Here's how the part is built. I have some questions about the finished solid (model axes, mm). A direction names the side the tool comes from. Round coordinates to 2 decimals unless told otherwise and drop trailing zeros. Loops run counter-clockwise (first coordinate to the right, second up) from the corner with the lowest first, then second, coordinate; pieces in that order, holes last. Notation, with made-up numbers: (1.25, -12.5) - (20.25, -12.5) arc R21 ccw to (20.25, -0.5) - close; hole circle Ø10 at (-20, 55.25). An arc over 180 degrees is marked (long way). Answer as a JSON object with one key per item and string values. Group by question number.
1) If I drill on line 1 along Y through (x, z) = (-11.5, -27); line 2 along Y through (x, z) = (7.5, 13); line 3 along X through (y, z) = (-6.5, -13.5), over which ranges is the centre line in solid material (lowest first)? Write a range as [from, to].
2) If we mould it in two halves opening along X, with no side actions, what happens to faces 1 (the face through (-15.825, -5, -20)), 2 (the face through (-6, -5, -30)), 3 (the face through (10, -24, -4)), 4 (the face through (-22, -26, -4))? For each: pulls with the +X half, pulls with the -X half, needs draft (parallel to the pull), parting line crosses it, or undercut.
3) I want a section at C-C, the plane y = -46. Please give me the cut outline in (x, z).
4) I want a section at D-D, the plane x = -6. Please give me the cut outline in (y, z).
5) I want a section at B-B, the plane x = -18. Please give me the cut outline in (y, z).
6) Which directions (+Z, -Z, +X, -X, +Y, -Y) give clear straight access to the entire face, cutting with the end or side of a thin tool? Please do faces 5 (the face through (6, -5, -27)), 6 (the face through (-2, -10, -20)), 7 (the face through (-6, -20, 2)).
7) Will these pins go through, and if not, where does the flat tip stop? P1, Ø6, axis at x = -4.5, y = -14.5, coming from the -Z side; P2, Ø5, axis at x = -1, y = -6, coming from the +Z side; P3, Ø8, axis at x = -7, z = -14.5, coming from the +Y side.
8) I want a section at A-A, the plane z = -19.5. Please give me the cut outline in (x, y) (3 decimals), then the cut area to 4 significant figures.
from build123d import *

# Parameters (mm, degrees)
F1_DEPTH = 50
F2_W     = 40
F2_H     = 28
F2_H_2   = 20
F3_DEPTH = 32.001
F4_SIZE  = 1


with BuildPart() as f1:
    # F0 (on Front) → F1 (new body)
    with BuildSketch(Plane.XZ):
        with BuildLine():
            Line((-22, 30), (-22, -30))
            Line((-22, -30), (-2, -30))
            Line((-2, -30), (-2, 9.9960947032))
            ThreePointArc((-2, 9.9960947032), (-8.25, 18), (-2, 26.0039052968))
            Line((-2, 26.0039052968), (-2, 30))
            Line((-2, 30), (-22, 30))
        make_face()
        with BuildLine():
            ThreePointArc((-15.825, -24.825), (-18, -27), (-20.175, -24.825))
            Line((-20.175, -24.825), (-20.175, -15.175))
            ThreePointArc((-20.175, -15.175), (-18, -13), (-15.825, -15.175))
            Line((-15.825, -15.175), (-15.825, -24.825))
        make_face(mode=Mode.SUBTRACT)
        with BuildLine():
            ThreePointArc((-3.825, -24.825), (-6, -27), (-8.175, -24.825))
            Line((-8.175, -24.825), (-8.175, -15.175))
            ThreePointArc((-8.175, -15.175), (-6, -13), (-3.825, -15.175))
            Line((-3.825, -15.175), (-3.825, -24.825))
        make_face(mode=Mode.SUBTRACT)
        with BuildLine():
            Line((-2, 9.9960947032), (-2, -30))
            Line((-2, -30), (10, -30))
            Line((10, -30), (10, 30))
            Line((10, 30), (-2, 30))
            Line((-2, 30), (-2, 26.0039052968))
            ThreePointArc((-2, 26.0039052968), (5.0775240029, 24.5024034018), (8.25, 18))
            ThreePointArc((8.25, 18), (5.0775240029, 11.4975965982), (-2, 9.9960947032))
        make_face()
        with BuildLine():
            Line((3.825, -24.825), (3.825, -15.175))
            ThreePointArc((3.825, -15.175), (6, -13), (8.175, -15.175))
            Line((8.175, -15.175), (8.175, -24.825))
            ThreePointArc((8.175, -24.825), (6, -27), (3.825, -24.825))
        make_face(mode=Mode.SUBTRACT)
    extrude(amount=F1_DEPTH)

    # F2 (on face) → F3 (cut, through all)
    with BuildSketch(Plane.YZ.offset(10)):
        with Locations((-20, 16)):
            Rectangle(F2_W, F2_H)
        with Locations((-30, -20)):
            Rectangle(F2_W, F2_H_2)
    extrude(amount=-F3_DEPTH, mode=Mode.SUBTRACT)

    # F4
    f4_edges = [f1.edges().sort_by_distance(p)[0] for p in [
        (10, -20, 2),
        (10, -40, 16),
        (10, -45, 30),
        (10, -50, 10),
        (10, -5, -30),
        (-6, -50, 30),
        (-22, -20, 2),
        (-22, -5, -30),
        (-22, -50, 10),
        (-22, -45, 30),
        (-22, -40, 16),
        (-6, -50, -10),
        (-6, -40, 30),
    ]]
    chamfer(f4_edges, length=F4_SIZE)


solid = f1.part
Outcome:
{
 "1": {"line 1": "[-10, 0]", "line 2": "[-50, -40]", "line 3": "[-22, -19.39], [-16.61, -7.39], [-4.61, 4.61], [7.39, 10]"},
 "2": {"face 1": "undercut", "face 2": "needs draft", "face 3": "pulls with the +X half", "face 4": "pulls with the -X half"},
 "3": {"outline": "(-22, -10) - (10, -10) - (10, 29) - (9, 30) - (-21, 30) - (-22, 29) - close; hole circle Ø16.5 at (0, 18)"},
 "4": {"outline": "(-50, -9) - (-49, -10) - (-10, -10) - (-10, -13) - (0, -13) - (0, 2) - (-40, 2) - (-40, 12.34) - (-50, 12.34) - close; (-50, 23.66) - (-40, 23.66) - (-40, 29) - (-41, 30) - (-49, 30) - (-50, 29) - close; (-10, -30) - (0, -30) - (0, -27) - (-10, -27) - close"},
 "5": {"outline": "(-50, -9) - (-49, -10) - (-10, -10) - (-10, -13) - (0, -13) - (0, 2) - (-40, 2) - (-40, 29) - (-41, 30) - (-49, 30) - (-50, 29) - close; (-10, -30) - (0, -30) - (0, -27) - (-10, -27) - close"},
 "6": {"face 5": "+Y, -Y", "face 6": "-Z, +X, -X, -Y", "face 7": "+Z, +X, -X, +Y"},
 "7": {"P1": "z = -10", "P2": "z = 2", "P3": "y = 0"},
 "8": {"outline": "(-22, -10) - (-20.175, -10) - (-20.175, 0) - (-22, 0) - close; (-15.825, -10) - (-8.175, -10) - (-8.175, 0) - (-15.825, 0) - close; (-3.825, -10) - (3.825, -10) - (3.825, 0) - (-3.825, 0) - close; (8.175, -10) - (10, -10) - (10, 0) - (8.175, 0) - close", "area": "189.5 mm^2"}
}
